Part model, mm, in its own coordinate system. Give positions to 0.01 mm unless a question says otherwise; leave off trailing zeros. Order: outer loops, then holes, each group sorted by start corner. A loop starts at its lowest first (then second) coordinate and runs counter-clockwise, first axis right, second up. Notation, with made-up numbers: M 80.5,-13 L 101.5,-13 A30 cw 101.5,19 Z; hole C -21,85.5 d6. An arc over 180 degrees is marked long. Answer as a JSON object with one key per item and string values.
from build123d import *

# Parameters (mm, degrees)
SKETCH1_W           = 609.6
SKETCH1_H           = 609.6
BOSS_EXTRUDE1_DEPTH = 12.7
SKETCH2_R           = 209.55
CUT_EXTRUDE1_DEPTH  = 13.7
SKETCH3_R           = 3
CUT_EXTRUDE2_DEPTH  = 13.7


with BuildPart() as part:
    # Sketch1 → Boss-Extrude1 (new body)
    with BuildSketch(Plane(origin=(0, 0, 0), x_dir=(1, 0, 0), z_dir=(0, 1, 0))):
        with Locations((254.294265396, -260.340726581)):
            Rectangle(SKETCH1_W, SKETCH1_H)
    extrude(amount=BOSS_EXTRUDE1_DEPTH)

    # Sketch2 → Cut-Extrude1 (cut, through all)
    with BuildSketch(Plane(origin=(0, 12.7, 0), x_dir=(1, 0, 0), z_dir=(0, 1, 0))):
        with Locations((254.294265396, -260.340726581)):
            Circle(SKETCH2_R)
    extrude(amount=-CUT_EXTRUDE1_DEPTH, mode=Mode.SUBTRACT)

    # Sketch3 → Cut-Extrude2 (cut, through all)
    with BuildSketch(Plane.XZ):
        with Locations((-37.805734604, 552.440726581)):
            Circle(SKETCH3_R)
        with Locations((546.394265396, 552.440726581)):
            Circle(SKETCH3_R)
        with Locations((546.394265396, -31.759273419)):
            Circle(SKETCH3_R)
        with Locations((-37.805734604, -31.759273419)):
            Circle(SKETCH3_R)
    extrude(amount=-CUT_EXTRUDE2_DEPTH, mode=Mode.SUBTRACT)


solid = part.part
1. Probe line 1 along Z through (x, y) = (248.5, 11.5); line 2 along Z through (x, y) = (448, 9); line 3 along X through (y, z) = (2.25, 359). List the from-to ranges inside material, lowest first.
Worked answers:
{"line 1": "z = -44.46 to 50.87, 469.81 to 565.14", "line 2": "z = -44.46 to 180.41, 340.27 to 565.14", "line 3": "x = -50.51 to 69.42, 439.17 to 559.09"}
2. Cut at C-C on y = 9.5. Give the cut face in (x, z).
Worked answers:
{"outline": "M -50.51,-44.46 L 559.09,-44.46 L 559.09,565.14 L -50.51,565.14 Z; hole C -37.81,-31.76 d6; hole C -37.81,552.44 d6; hole C 254.29,260.34 d419.1; hole C 546.39,-31.76 d6; hole C 546.39,552.44 d6"}
3. Two-plate mould, pull along Z, no slides. Class faces 1 (the flat face through (182, 12.7, 53)), 2 (the cylindrical face through (447.865, 6.439, 340.6)): +Z half, -Z half, draft (parallel to the pull), parting line (faces both ways), or undercut.
Worked answers:
{"face 1": "draft", "face 2": "undercut"}
4. Cut at A-A on x = 127. Give the cut face in (y, z).
Worked answers:
{"outline": "M 0,-44.46 L 12.7,-44.46 L 12.7,93.89 L 0,93.89 Z; M 0,426.8 L 12.7,426.8 L 12.7,565.14 L 0,565.14 Z"}
5. Cut at B-B on z = 69. Give the cut face in (x, y).
Worked answers:
{"outline": "M -50.51,0 L 168.85,0 L 168.85,12.7 L -50.51,12.7 Z; M 339.73,0 L 559.09,0 L 559.09,12.7 L 339.73,12.7 Z"}
